Model file for the job. Use its own axes, mm. Face numbers are marked on the shaded views. A direction names the side the tool comes from. Coordinates: 2 decimals unless noted, no trailing zeros. Write each loop counter-clockwise with the first axis right and the second up, starting at its lowest first coordinate (ties: lowest second). Pieces come first, ordered by that corner, then holes.
Q1. Pull direction X, two halves, no side cores. Call the marked faces 1, 2 and 3: released by +X, released by -X, zero draft, split by the parting line, or undercut.
Q2. Band-saw the part on B-B, the plane z = 27. Write the cut outline in (x, y).
Q3. Band-saw the part on D-D, the plane x = -15. Write the cut outline in (y, z), plus the area to 3 significant figures.
Q4. Which spindle directions (+Z, -Z, +X, -X, +Y, -Y) get a long thin tool onto all of the face, cutting with end or side? Do the marked faces 4, 5, 6 and 7. Say none if no direction does.
Q5. Pin check, flat tips, straight feed: P1, Ø8, axis at x = 22, z = 15, coming from the +Y side; P2, Ø10, axis at x = -4.5, y = -74, coming from the -Z side; P3, Ø5, axis at x = -3, z = 27.5, coming from the -Y side; P4, Ø6.5, axis at x = -2, z = 15, coming from the -Y side (3 decimals). Stop position of each tip, or through.
Q6. Band-saw the part on C-C, the plane y = -107.85. Write the cut outline in (x, z), plus the area to 3 significant figures.
Q7. Drill centre lines: probe 1 along Y at (x, z) = (-10, 3.9); probe 2 along Z at (x, y) = (-23.9, -55.05); probe 3 along X at (y, z) = (-101, 8). Where is each one in solid material? Low to high.
Q8. Band-saw the part on A-A, the plane y = -55.05. Write the cut outline in (x, z).
from build123d import *

# Parameters (mm, degrees)
BOSS_EXTRU_1_DEPTH      = 10
ENL_V_MAT_EXTRU_1_REACH = 118.172
ESQUISSE2_R             = 1.75
ESQUISSE4_R             = 3.5
ENL_V_MAT_EXTRU_2_DEPTH = 4
ESQUISSE5_W             = 50
ESQUISSE5_H             = 38
BOSS_EXTRU_2_DEPTH      = 14.4
ENL_V_MAT_EXTRU_3_REACH = 55.304
ESQUISSE6_R             = 1.5
ESQUISSE7_R             = 3
ENL_V_MAT_EXTRU_4_DEPTH = 9.4
CHANFREIN1_SIZE         = 10
CHANFREIN2_SIZE         = 28
CHANFREIN2_SIZE_2       = 10
BOSS_EXTRU_3_DEPTH      = 5
ESQUISSE9_W             = 38
ESQUISSE9_H             = 28.6
BOSS_EXTRU_4_DEPTH      = 2.5
CHANFREIN3_SIZE         = 5
ENL_V_MAT_EXTRU_5_REACH = 134.155
ESQUISSE10_R            = 1.5
ESQUISSE11_R            = 3
ENL_V_MAT_EXTRU_6_DEPTH = 2.5


# Some blends are built 0.0001 mm under size
with BuildPart() as part:
    # Esquisse1 → Boss.-Extru.1 (new body)
    with BuildSketch(Plane.XY):
        with BuildLine():
            Line((-20, -112.231902773), (-20, -91.7))
            Line((-20, -91.7), (20, -91.7))
            Line((20, -91.7), (20, -112.231902773))
            ThreePointArc((20, -112.231902773), (0, -114), (-20, -112.231902773))
        make_face()
    extrude(amount=BOSS_EXTRU_1_DEPTH)

    # Esquisse2 → Enlèv. mat.-Extru.1 (cut, up to next)
    with BuildSketch(Plane.XY.offset(10), mode=Mode.PRIVATE) as enl_v_mat_extru_1_sk1:
        with Locations((-10, -97.85)):
            Circle(ESQUISSE2_R)
    enl_v_mat_extru_1_tool1 = extrude(enl_v_mat_extru_1_sk1.sketch, amount=-ENL_V_MAT_EXTRU_1_REACH, mode=Mode.PRIVATE) & part.part
    # Esquisse2 → Enlèv. mat.-Extru.1 (cut, up to next)
    with BuildSketch(Plane.XY.offset(10), mode=Mode.PRIVATE) as enl_v_mat_extru_1_sk2:
        with Locations((-10, -107.85)):
            Circle(ESQUISSE2_R)
    enl_v_mat_extru_1_tool2 = extrude(enl_v_mat_extru_1_sk2.sketch, amount=-ENL_V_MAT_EXTRU_1_REACH, mode=Mode.PRIVATE) & part.part
    # Esquisse2 → Enlèv. mat.-Extru.1 (cut, up to next)
    with BuildSketch(Plane.XY.offset(10), mode=Mode.PRIVATE) as enl_v_mat_extru_1_sk3:
        with Locations((10, -97.85)):
            Circle(ESQUISSE2_R)
    enl_v_mat_extru_1_tool3 = extrude(enl_v_mat_extru_1_sk3.sketch, amount=-ENL_V_MAT_EXTRU_1_REACH, mode=Mode.PRIVATE) & part.part
    # Esquisse2 → Enlèv. mat.-Extru.1 (cut, up to next)
    with BuildSketch(Plane.XY.offset(10), mode=Mode.PRIVATE) as enl_v_mat_extru_1_sk4:
        with Locations((10, -107.85)):
            Circle(ESQUISSE2_R)
    enl_v_mat_extru_1_tool4 = extrude(enl_v_mat_extru_1_sk4.sketch, amount=-ENL_V_MAT_EXTRU_1_REACH, mode=Mode.PRIVATE) & part.part
    add(enl_v_mat_extru_1_tool1.solids().sort_by_distance((-10, -97.85, 10))[0], mode=Mode.SUBTRACT)
    add(enl_v_mat_extru_1_tool2.solids().sort_by_distance((-10, -107.85, 10))[0], mode=Mode.SUBTRACT)
    add(enl_v_mat_extru_1_tool3.solids().sort_by_distance((10, -97.85, 10))[0], mode=Mode.SUBTRACT)
    add(enl_v_mat_extru_1_tool4.solids().sort_by_distance((10, -107.85, 10))[0], mode=Mode.SUBTRACT)

    # Esquisse4 → Enlèv. mat.-Extru.2 (cut)
    with BuildSketch(Plane.XY.offset(10)):
        with Locations((-10, -97.85)):
            Circle(ESQUISSE4_R)
        with Locations((10, -97.85)):
            Circle(ESQUISSE4_R)
        with Locations((10, -107.85)):
            Circle(ESQUISSE4_R)
        with Locations((-10, -107.85)):
            Circle(ESQUISSE4_R)
    extrude(amount=-ENL_V_MAT_EXTRU_2_DEPTH, mode=Mode.SUBTRACT)

    # Esquisse5 → Boss.-Extru.2 (add)
    with BuildSketch(Plane(origin=(0, -91.7, 0), x_dir=(1, 0, 0), z_dir=(0, 1, 0))):
        with Locations((5, -19)):
            Rectangle(ESQUISSE5_W, ESQUISSE5_H)
    extrude(amount=BOSS_EXTRU_2_DEPTH)

    # Esquisse6 → Enlèv. mat.-Extru.3 (cut, up to next)
    with BuildSketch(Plane.XZ.offset(91.7), mode=Mode.PRIVATE) as enl_v_mat_extru_3_sk1:
        with Locations(Location((-2, 27, 0), (0, 0, 270))):
            Circle(ESQUISSE6_R)
    enl_v_mat_extru_3_tool1 = extrude(enl_v_mat_extru_3_sk1.sketch, amount=-ENL_V_MAT_EXTRU_3_REACH, mode=Mode.PRIVATE) & part.part
    # Esquisse6 → Enlèv. mat.-Extru.3 (cut, up to next)
    with BuildSketch(Plane.XZ.offset(91.7), mode=Mode.PRIVATE) as enl_v_mat_extru_3_sk2:
        with Locations(Location((22, 27, 0), (0, 0, 270))):
            Circle(ESQUISSE6_R)
    enl_v_mat_extru_3_tool2 = extrude(enl_v_mat_extru_3_sk2.sketch, amount=-ENL_V_MAT_EXTRU_3_REACH, mode=Mode.PRIVATE) & part.part
    # Esquisse6 → Enlèv. mat.-Extru.3 (cut, up to next)
    with BuildSketch(Plane.XZ.offset(91.7), mode=Mode.PRIVATE) as enl_v_mat_extru_3_sk3:
        with Locations(Location((-2, 15, 0), (0, 0, 270))):
            Circle(ESQUISSE6_R)
    enl_v_mat_extru_3_tool3 = extrude(enl_v_mat_extru_3_sk3.sketch, amount=-ENL_V_MAT_EXTRU_3_REACH, mode=Mode.PRIVATE) & part.part
    # Esquisse6 → Enlèv. mat.-Extru.3 (cut, up to next)
    with BuildSketch(Plane.XZ.offset(91.7), mode=Mode.PRIVATE) as enl_v_mat_extru_3_sk4:
        with Locations(Location((22, 15, 0), (0, 0, 270))):
            Circle(ESQUISSE6_R)
    enl_v_mat_extru_3_tool4 = extrude(enl_v_mat_extru_3_sk4.sketch, amount=-ENL_V_MAT_EXTRU_3_REACH, mode=Mode.PRIVATE) & part.part
    add(enl_v_mat_extru_3_tool1.solids().sort_by_distance((-2, -91.7, 27))[0], mode=Mode.SUBTRACT)
    add(enl_v_mat_extru_3_tool2.solids().sort_by_distance((22, -91.7, 27))[0], mode=Mode.SUBTRACT)
    add(enl_v_mat_extru_3_tool3.solids().sort_by_distance((-2, -91.7, 15))[0], mode=Mode.SUBTRACT)
    add(enl_v_mat_extru_3_tool4.solids().sort_by_distance((22, -91.7, 15))[0], mode=Mode.SUBTRACT)

    # Esquisse7 → Enlèv. mat.-Extru.4 (cut)
    with BuildSketch(Plane.XZ.offset(91.7)):
        with Locations(Location((-2, 27, 0), (0, 0, 270))):
            Circle(ESQUISSE7_R)
        with Locations(Location((22, 27, 0), (0, 0, 270))):
            Circle(ESQUISSE7_R)
        with Locations(Location((22, 15, 0), (0, 0, 270))):
            Circle(ESQUISSE7_R)
        with Locations(Location((-2, 15, 0), (0, 0, 270))):
            Circle(ESQUISSE7_R)
    extrude(amount=-ENL_V_MAT_EXTRU_4_DEPTH, mode=Mode.SUBTRACT)

    # Chanfrein1
    chanfrein1_edges = [part.edges().sort_by_distance(p)[0] for p in [
        (30, -84.5, 0),
    ]]
    chamfer(chanfrein1_edges, length=CHANFREIN1_SIZE)

    # Chanfrein2
    # the kernel refuses this chamfer: 28, 10 mm, written as the material it takes off along each edge
    with BuildSketch(Plane(origin=(102.642981969, -91.7, 38), x_dir=(0, -0.01296397650632004, -0.9999159641255577), z_dir=(-1, 0, 0))) as chanfrein2_piece_1:
        Polygon((CHANFREIN2_SIZE * 0.999915964126, -CHANFREIN2_SIZE * 0.0129639765063), (-CHANFREIN2_SIZE_2 * 0.0129639765063, -CHANFREIN2_SIZE_2 * 0.999915964126), (0, 0), align=None)
    extrude(amount=195.285963938, mode=Mode.SUBTRACT)

    # Esquisse8 → Boss.-Extru.3 (add)
    with BuildSketch(Plane.ZY.offset(20)):
        Polygon((10, -91.7), (0, -91.7), (0, -48.7), (38, -48.7), (38, -81.7), align=None)
    extrude(amount=BOSS_EXTRU_3_DEPTH)

    # Esquisse9 → Boss.-Extru.4 (add)
    with BuildSketch(Plane(origin=(-20, 0, 0), x_dir=(0, 0, -1), z_dir=(1, 0, 0))):
        with Locations((-19, -63)):
            Rectangle(ESQUISSE9_W, ESQUISSE9_H)
    extrude(amount=BOSS_EXTRU_4_DEPTH)

    # Chanfrein3
    chanfrein3_edges = [part.edges().sort_by_distance(p)[0] for p in [
        (-20, -91.7, 5),
    ]]
    chamfer(chanfrein3_edges, length=CHANFREIN3_SIZE - 0.0001)  # a hair under: the kernel refuses the full size

    # Esquisse10 → Enlèv. mat.-Extru.5 (cut, up to next)
    with BuildSketch(Plane.ZY.offset(25), mode=Mode.PRIVATE) as enl_v_mat_extru_5_sk1:
        with Locations(Location((15, -55.05, 0), (0, 0, 270))):
            Circle(ESQUISSE10_R)
    enl_v_mat_extru_5_tool1 = extrude(enl_v_mat_extru_5_sk1.sketch, amount=-ENL_V_MAT_EXTRU_5_REACH, mode=Mode.PRIVATE) & part.part
    # Esquisse10 → Enlèv. mat.-Extru.5 (cut, up to next)
    with BuildSketch(Plane.ZY.offset(25), mode=Mode.PRIVATE) as enl_v_mat_extru_5_sk2:
        with Locations(Location((15, -71.05, 0), (0, 0, 270))):
            Circle(ESQUISSE10_R)
    enl_v_mat_extru_5_tool2 = extrude(enl_v_mat_extru_5_sk2.sketch, amount=-ENL_V_MAT_EXTRU_5_REACH, mode=Mode.PRIVATE) & part.part
    add(enl_v_mat_extru_5_tool1.solids().sort_by_distance((-25, -55.05, 15))[0], mode=Mode.SUBTRACT)
    add(enl_v_mat_extru_5_tool2.solids().sort_by_distance((-25, -71.05, 15))[0], mode=Mode.SUBTRACT)

    # Esquisse11 → Enlèv. mat.-Extru.6 (cut)
    with BuildSketch(Plane.ZY.offset(25)):
        with Locations(Location((15, -55.05, 0), (0, 0, 270))):
            Circle(ESQUISSE11_R)
        with Locations(Location((15, -71.05, 0), (0, 0, 270))):
            Circle(ESQUISSE11_R)
    extrude(amount=-ENL_V_MAT_EXTRU_6_DEPTH, mode=Mode.SUBTRACT)


solid = part.part
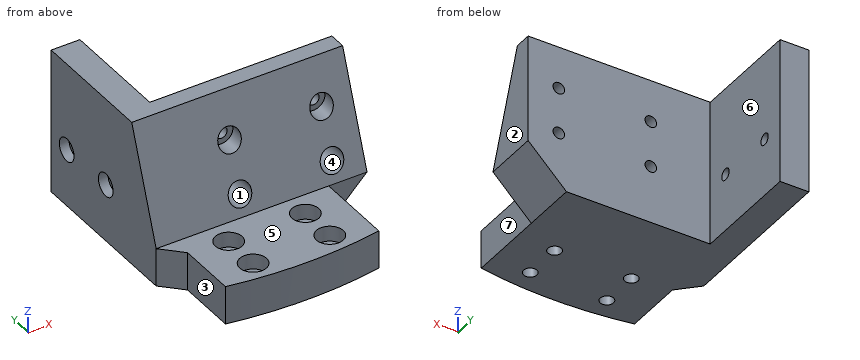
Answer sheet:
1. face 1: undercut
1. face 2: released by +X
1. face 3: released by -X
2. outline: (-25, -85.63) - (-5, -85.63) - (-5, -82.3) - (-3.5, -82.3) - (-3.5, -77.3) - (-17.5, -77.3) - (-17.5, -48.7) - (-25, -48.7) - close; (-0.5, -82.3) - (1, -82.3) - (1, -85.63) - (19, -85.63) - (19, -82.3) - (20.5, -82.3) - (20.5, -77.3) - (-0.5, -77.3) - close; (23.5, -82.3) - (25, -82.3) - (25, -85.63) - (30, -85.63) - (30, -77.3) - (23.5, -77.3) - close
3. outline: (-113.01, 0) - (-77.3, 0) - (-77.3, 38) - (-81.7, 38) - (-91.7, 10) - (-113.01, 10) - close
3. area: 620 mm2
4. face 4: -Y
4. face 5: +Z, +X, -X, -Y
4. face 6: +Z, -Z, +X, +Y
4. face 7: +Z, -Z, +X, -Y
5. P1: stops at y = -77.3
5. P2: stops at z = 0
5. P3: stops at y = -86.11
5. P4: stops at y = -91.075
6. outline: (-20, 0) - (-11.75, 0) - (-11.75, 6) - (-13.5, 6) - (-13.5, 10) - (-20, 10) - close; (-8.25, 0) - (8.25, 0) - (8.25, 6) - (6.5, 6) - (6.5, 10) - (-6.5, 10) - (-6.5, 6) - (-8.25, 6) - close; (11.75, 0) - (20, 0) - (20, 10) - (13.5, 10) - (13.5, 6) - (11.75, 6) - close
6. area: 302 mm2
7. probe 1: y = -113.56 to -109.6, -106.1 to -99.6, -96.1 to -77.3
7. probe 2: z = 0 to 12, 18 to 38
7. probe 3: x = -20 to -11.53, -8.47 to 8.47, 11.53 to 20
8. outline: (-25, 0) - (-17.5, 0) - (-17.5, 13.5) - (-22.5, 13.5) - (-22.5, 12) - (-25, 12) - close; (-25, 18) - (-22.5, 18) - (-22.5, 16.5) - (-17.5, 16.5) - (-17.5, 38) - (-25, 38) - close
